```python
from build123d import *

# Parameters (mm, degrees)
F1_DEPTH    = 10
F2_R        = 3.25
F3_DEPTH    = 10
F4_T1_DEPTH = 61.4336597593


# Not quite as in the source:
# - a fillet or chamfer that OpenCascade refuses, or shapes differently, is made with other operations: its cross-section is extruded or revolved along the edge and cut away or added


with BuildPart() as f1:
    # F0 (on Top) → F1 (new body)
    with BuildSketch(Plane.XY):
        with BuildLine():
            Line((20, 20), (-80, 20))
            Line((-80, 20), (-80, -20))
            Line((-80, -20), (20, -20))
            ThreePointArc((20, -20), (40, 0), (20, 20))
        make_face()
        with BuildLine():
            ThreePointArc((20, 15), (35, 0), (20, -15))
            Line((20, -15), (7, -15))
            ThreePointArc((7, -15), (-8, 0), (7, 15))
            Line((7, 15), (20, 15))
        make_face(mode=Mode.SUBTRACT)
    extrude(amount=F1_DEPTH)

    # F2 (on face) → F3 (cut)
    with BuildSketch(Plane(origin=(-80, 0, 0), x_dir=(0, -1, 0), z_dir=(-1, 0, 0))):
        with Locations((-15, 5)):
            Circle(F2_R)
        with Locations((15, 5)):
            Circle(F2_R)
    extrude(amount=-F3_DEPTH, mode=Mode.SUBTRACT)

    # F4: chamfer of 10 on 2 edges, made by hand

    # F4_s2 → F4_t1 (cut)
    with BuildSketch(Plane.XY.offset(-25.7168298797)):
        Polygon((-70, 20), (-80, 10), (-80, 20), align=None)
        Polygon((-80, -10), (-70, -20), (-80, -20), align=None)
    extrude(amount=F4_T1_DEPTH, mode=Mode.SUBTRACT)


solid = f1.part
```
The listing builds one solid part. Answer for the finished solid, in the listing's coordinates (mm). A direction names the side the tool comes from. Give positions to 0.01 mm unless a question says otherwise; leave off trailing zeros. Order: outer loops, then holes, each group sorted by start corner. A loop starts at its lowest first (then second) coordinate and runs counter-clockwise, first axis right, second up. Notation, with made-up numbers: (-35, 84.5) -> (-3, 84.5) arc R24 cw to (-3, 95.5) -> close; hole circle Ø6 at (-19.5, 26). An arc over 180 degrees is marked (long way). Answer as a JSON object with one key per item and string values. Group by question number.
Item 1: The part is cut by section C-C on x = 1. Write down the section's boundary in (y, z).
Item 2: Determine the mould class of faces 1 (the flat face through (-70, -15, 5)), 2 (the cylindrical face through (-8, 0, 5)), 3 (the cylindrical face through (-73.319, -11.753, 5.143)), 4 (the flat face through (-34, 0, 10)) for opening direction Z: pulls with the +Z half, pulls with the -Z half, needs draft (parallel to the pull), parting line crosses it, or undercut.
Item 3: A tool of negligible diameter and unlimited length cuts with its end or side. For faces 5 (the cylindrical face through (35, 0, 5)), 6 (the cylindrical face through (40, 0, 5)), 7 (the cylindrical face through (-73.27, 11.9, 5.98)), from which of +Z, -Z, +X, -X, +Y, -Y can it reach the whole face along a straight path? Write none if from no direction.
Item 4: Flat-ended cylindrical pins translate along their axes: pin 1 (3 mm diameter, centred on y = 15.5, z = 4.5, fed in from -X); pin 2 (1.5 mm diameter, centred on y = 0, z = 7.5, fed in from +X); pin 3 (4 mm diameter, centred on y = -7, z = 1, fed in from +X). Find the tip coordinate at first contact, or state that the pin passes through.
Item 5: The part is cut by section B-B on z = 3.75. Write down the section's boundary in (x, y), and give its area (3 significant figures).
Item 6: The part is cut by section A-A on y = 0. Write down the section's boundary in (x, z), and give its area (3 significant figures).
Item 7: Consider L1, parallel to Z at x = -74, y = -15; L2, parallel to Y at x = 10.5, z = 5; L3, parallel to Y at x = 5, z = 2. Determine where each line is inside the solid, lowest interval first. Write a range as from..to.
Result set:
{
 "1": {"outline": "(-20, 0) -> (-13.75, 0) -> (-13.75, 10) -> (-20, 10) -> close; (13.75, 0) -> (20, 0) -> (20, 10) -> (13.75, 10) -> close"},
 "2": {"face 1": "undercut", "face 2": "needs draft", "face 3": "undercut", "face 4": "pulls with the +Z half"},
 "3": {"face 5": "+Z, -Z", "face 6": "+Z, -Z, +X", "face 7": "-X"},
 "4": {"pin 1": "x = -70", "pin 2": "x = 40", "pin 3": "x = 39.36"},
 "5": {"outline": "(-80, -10) -> (-78, -12) -> (-70, -12) -> (-70, -18) -> (-72, -18) -> (-70, -20) -> (20, -20) arc R20 ccw to (20, 20) -> (-70, 20) -> (-72, 18) -> (-70, 18) -> (-70, 12) -> (-78, 12) -> (-80, 10) -> close; hole (7, -15) -> (20, -15) arc R15 ccw to (20, 15) -> (7, 15) arc R15 ccw to start", "area": "3,370 mm²"},
 "6": {"outline": "(-80, 0) -> (-8, 0) -> (-8, 10) -> (-80, 10) -> close; (35, 0) -> (40, 0) -> (40, 10) -> (35, 10) -> close", "area": "770 mm²"},
 "7": {"L1": "0..1.75, 8.25..10", "L2": "-20..-15, 15..20", "L3": "-20..-14.87, 14.87..20"}
}
